Source: CAD feature listing. Evaluate the final solid. Frame: model axes, mm. A direction names the side the tool comes from. Give positions to 0.01 mm unless a question says otherwise; leave off trailing zeros. Loops run counter-clockwise (first coordinate to the right, second up) from the corner with the lowest first, then second, coordinate; pieces in that order, holes last. Notation, with made-up numbers: M -32,-33 L -2,-33 A23 cw -2,-4 Z; hole C 23,5.25 d6. An arc over 180 degrees is marked long. Answer in a Markdown table with one row per item.
```python
from build123d import *

# Parameters (mm, degrees)
F2_SIZE  = 1
F3_R     = 1
F5_W     = 7.37243
F5_H     = 8.687595
F6_DEPTH = 1


with BuildPart() as f1:
    # F0 (on Front) → F1 (revolve)
    with BuildSketch(Plane.XZ):
        Polygon((-50, 10), (-50, 0), (50, 0), (50, 10), (35, 10), (35, 15), (-35, 15), (-35, 10), align=None)
    revolve(axis=Axis((0, 0, 0), (-1, 0, 0)))

    # F2
    f2_edges = [f1.edges().sort_by_distance(p)[0] for p in [
        (-50, 0, -10),
        (50, 0, -10),
    ]]
    chamfer(f2_edges, length=F2_SIZE)

    # F3
    f3_edges = [f1.edges().sort_by_distance(p)[0] for p in [
        (-35, 0, -10),
        (35, 0, -10),
    ]]
    fillet(f3_edges, radius=F3_R)

    # F5 (on offset) → F6 (cut)
    with BuildSketch(Plane.XY.offset(10)):
        with Locations((-42.681136, 0.846396)):
            Rectangle(F5_W, F5_H)
    extrude(amount=-F6_DEPTH, mode=Mode.SUBTRACT)


solid = f1.part
```
1) Pin query (flat end, axial travel): pin 1 Ø3 at (x, z) = (36, -1.5) entering from -Y; pin 2 Ø12 at (x, y) = (-10, 8) entering from -Z; pin 3 Ø8 at (x, y) = (-43, 1) entering from +Z. Return the tip coordinate at first contact, or that it passes through.
Reply:
| item | result |
|---|---|
| pin 1 | stops at y = -15 |
| pin 2 | stops at z = -14.87 |
| pin 3 | stops at z = 10 |
2) Pull-direction query (X, two-part tool) for faces 4 (the flat face through (-35, 10, -5)), 5 (the flat face through (50, 0, 0)), 6 (the cylindrical face through (42.41, -9.76, -2.17)), 7 (the flat face through (-43, 0, 9)); classes: released by +X, released by -X, zero draft, split by the parting line, or undercut.
Reply:
| item | result |
|---|---|
| face 4 | released by -X |
| face 5 | released by +X |
| face 6 | zero draft |
| face 7 | undercut |
3) Section D-D, the plane x = 39. Return loops of the section in (y, z).
Reply:
| item | result |
|---|---|
| outline | C 0,0 d20 |
4) Section C-C, the plane x = 8. Return loops of the section in (y, z), then the cut area to 3 significant figures.
Reply:
| item | result |
|---|---|
| outline | C 0,0 d30 |
| area | 707 mm² |
5) Section B-B, the plane z = 0. Return loops of the section in (x, y).
Reply:
| item | result |
|---|---|
| outline | M -50,-9 L -49,-10 L -36,-10 A1 cw -35,-11 L -35,-15 L 35,-15 L 35,-11 A1 cw 36,-10 L 49,-10 L 50,-9 L 50,9 L 49,10 L 36,10 A1 cw 35,11 L 35,15 L -35,15 L -35,11 A1 cw -36,10 L -49,10 L -50,9 Z |
6) Material intervals for L1, parallel to X at y = 9.75, z = 9; L2, parallel to Z at x = 25, y = -10.5; L3, parallel to Z at x = -14.5, y = 1.5, sorted ascending.
Reply:
| item | result |
|---|---|
| L1 | x = -35 to 35 |
| L2 | z = -10.71 to 10.71 |
| L3 | z = -14.92 to 14.92 |
7) Set-up query: faces 1 (the flat face through (35, 10, 5)), 2 (the cylindrical face through (-0.49, 0.66, -14.985)), 3 (the cylindrical face through (-43, -6, -8)). Return all of +Z, -Z, +X, -X, +Y, -Y with unobstructed straight access to the full face (end or side cutting, diameter ignored); none if empty.
Reply:
| item | result |
|---|---|
| face 1 | +X |
| face 2 | +X, -X |
| face 3 | -X |
8) Section A-A, the plane y = 0. Return loops of the section in (x, z), then the cut area to 3 significant figures.
Reply:
| item | result |
|---|---|
| outline | M -50,-9 L -49,-10 L -36,-10 A1 cw -35,-11 L -35,-15 L 35,-15 L 35,-11 A1 cw 36,-10 L 49,-10 L 50,-9 L 50,9 L 49,10 L 36,10 A1 cw 35,11 L 35,15 L -35,15 L -35,11 A1 cw -36,10 L -38.99,10 L -38.99,9 L -46.37,9 L -46.37,10 L -49,10 L -50,9 Z |
| area | 2,690 mm² |
